```python
from build123d import *

# Parameters (mm, degrees)
SKETCH1_R           = 8
BOSS_EXTRUDE1_DEPTH = 12
BOSS_EXTRUDE2_START = 8
SKETCH2_R           = 8
BOSS_EXTRUDE2_DEPTH = 12
BOSS_EXTRUDE3_START = -20
SKETCH2_3_R         = 8
BOSS_EXTRUDE3_DEPTH = 12
SKETCH3_R           = 8
BOSS_EXTRUDE4_DEPTH = 12


with BuildPart() as part:
    # Sketch1 → Boss-Extrude1 (new body)
    with BuildSketch(Plane(origin=(0, 0, 0), x_dir=(1, 0, 0), z_dir=(0, 1, 0))):
        with BuildLine():
            Line((20, 0), (-20, 0))
            Line((-20, 0), (-20, -60))
            ThreePointArc((-20, -60), (0, -80), (20, -60))
            Line((20, -60), (20, 0))
        make_face()
        with Locations(Location((0, -60, 0), (0, 0, 270))):
            Circle(SKETCH1_R, mode=Mode.SUBTRACT)
    extrude(amount=BOSS_EXTRUDE1_DEPTH)

    # Sketch2 → Boss-Extrude2 (add)
    with BuildSketch(Plane(origin=(0, 0, 0), x_dir=(0, 0, -1), z_dir=(1, 0, 0)).offset(BOSS_EXTRUDE2_START)):
        with BuildLine():
            Line((-40, 12), (0, 12))
            Line((0, 12), (0, 32))
            ThreePointArc((0, 32), (-20, 52), (-40, 32))
            Line((-40, 32), (-40, 12))
        make_face()
        with Locations((-20, 32)):
            Circle(SKETCH2_R, mode=Mode.SUBTRACT)
    extrude(amount=BOSS_EXTRUDE2_DEPTH)

    # Sketch2_3 → Boss-Extrude3 (add)
    with BuildSketch(Plane(origin=(0, 0, 0), x_dir=(0, 0, -1), z_dir=(1, 0, 0)).offset(BOSS_EXTRUDE3_START)):
        with BuildLine():
            Line((-40, 12), (0, 12))
            Line((0, 12), (0, 32))
            ThreePointArc((0, 32), (-20, 52), (-40, 32))
            Line((-40, 32), (-40, 12))
        make_face()
        with Locations((-20, 32)):
            Circle(SKETCH2_3_R, mode=Mode.SUBTRACT)
    extrude(amount=BOSS_EXTRUDE3_DEPTH)

    # Sketch3 → Boss-Extrude4 (add)
    with BuildSketch(Plane.XY):
        with BuildLine():
            Line((20, 0), (-20, 0))
            Line((-20, 0), (-20, -28))
            ThreePointArc((-20, -28), (-0.013931924, -47.986068076), (19.972136151, -28))
            Line((19.972136151, -28), (20, 0))
        make_face()
        with Locations((-0.013931924, -28)):
            Circle(SKETCH3_R, mode=Mode.SUBTRACT)
    extrude(amount=BOSS_EXTRUDE4_DEPTH)


solid = part.part
```
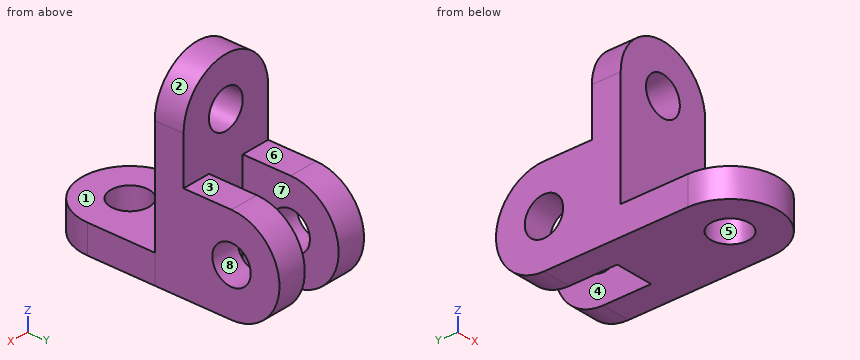
Part model, mm, in its own coordinate system. Face numbers are marked on the shaded views. A direction names the side the tool comes from. Coordinates: 2 decimals unless noted, no trailing zeros. Write each loop counter-clockwise with the first axis right and the second up, starting at its lowest first coordinate (ties: lowest second). Pieces come first, ordered by that corner, then holes.
Item 1: Probe line 1 (Y direction, x = 12.75, z = 20); line 2 (X direction, y = 27.5, z = 30); line 3 (Y direction, x = 15, z = 65.5). List the from-to ranges inside material, lowest first.
Item 2: Which spindle directions (+Z, -Z, +X, -X, +Y, -Y) get a long thin tool onto all of the face, cutting with end or side? Do the marked faces 1, 2, 3, 4 and 5. Say none if no direction does.
Item 3: Mould opens along Z. For the marked faces 6, 7 and 8 say: released by +Z, released by -Z, zero draft, split by the parting line, or undercut.
Item 4: Slice it at C-C (x = 6.5). Write the cut outline in (y, z).
Item 5: Pin check, flat tips, straight feed: pin 1 (9.5 mm diameter, centred on x = -11.5, y = 26.5, fed in from +Z); pin 2 (10 mm diameter, centred on x = -9, z = 54.5, fed in from +Y); pin 3 (1.5 mm diameter, centred on y = -12, z = 12, fed in from +X); pin 4 (13 mm diameter, centred on y = 32, z = 20, fed in from -X). Stop position of each tip, or through.
Item 6: Slice it at A-A (y = 4.5). Write the cut outline in (x, z).
Item 7: Slice it at B-B (z = 20). Write the cut outline in (x, y).
Item 8: Slice it at D-D (y = 15). Write the cut outline in (x, z).
Results found:
1. line 1: y = 0 to 24, 40 to 52
1. line 2: x = -20 to -8, 8 to 20
1. line 3: y = 0 to 12
2. face 1: +Z, +X, -X, -Y
2. face 2: +Z, +Y, -Y
2. face 3: +Z, +X, -X, +Y
2. face 4: +Z, -Z, +Y
2. face 5: +Z, -Z
3. face 6: released by +Z
3. face 7: zero draft
3. face 8: undercut
4. outline: (-46.89, 0) - (-32.64, 0) - (-32.64, 12) - (-46.89, 12) - close; (-23.36, 0) - (12, 0) - (12, 55.34) - (0, 55.34) - (0, 12) - (-23.36, 12) - close; (0, 64.66) - (12, 64.66) - (12, 78.91) - (0, 78.91) - close
5. pin 1: stops at z = 40
5. pin 2: stops at y = 12
5. pin 3: stops at x = 19.99
5. pin 4: passes through
6. outline: (-20, 0) - (20, 0) - (20, 60) arc R20 ccw to (-20, 60) - close; hole circle Ø16 at (0, 60)
7. outline: (-20, 0) - (20, 0) - (20, 24) - (8, 24) - (8, 12) - (-8, 12) - (-8, 24) - (-20, 24) - close; (-20, 40) - (-8, 40) - (-8, 52) - (-20, 52) - close; (8, 40) - (20, 40) - (20, 52) - (8, 52) - close
8. outline: (-20, 0) - (-8, 0) - (-8, 40) - (-20, 40) - close; (8, 0) - (20, 0) - (20, 40) - (8, 40) - close
